The listing builds one solid part. Answer for the finished solid, in the listing's coordinates (mm). A direction names the side the tool comes from. Give positions to 0.01 mm unless a question says otherwise; leave off trailing zeros. Loops run counter-clockwise (first coordinate to the right, second up) from the corner with the lowest first, then second, coordinate; pieces in that order, holes last. Notation, with made-up numbers: M 63.5,-14.5 L 76.5,-14.5 A7 cw 76.5,-10.5 Z; hole C 14.5,61 d3. An arc over 180 degrees is marked long. Use one line per item in the form item = value. Start each with the question number.
1. The part is cut by section A-A (x = 0). Write down the section's boundary in (y, z), and give its area (3 significant figures).
2. This flat-tipped pin is pushed along its axis until it touches: pin 1 Ø2 at (x, z) = (0, 0) entering from +Y. Where does it stop, or does it pass through?
3. The part is cut by section D-D (x = -1.5). Write down the section's boundary in (y, z), and give its area (3 significant figures).
4. Straight lines are drawn through the part: line 1 (Z direction, x = 0, y = 0.7); line 2 (Y direction, x = 0.5, z = 3); line 3 (Z direction, x = -1, y = 1.45). For each, find the intervals that lie inside material, in ascending order. Write a range as from..to.
5. The mould has two halves that part along X. Classify faces 3 (the face through (-1, 1, 0)), 4 (the face through (-5.5, 1.5, -0.1)), 5 (the face through (0, 0, -1)): released by +X, released by -X, zero draft, split by the parting line, or undercut.
6. The part is cut by section C-C (y = 0.65). Write down the section's boundary in (x, z), and give its area (3 significant figures).
7. For faces 1 (the face through (0, 1, -5)), 2 (the face through (-2.373, 2.014, -3.095)), determine the directions among +Z, -Z, +X, -X, +Y, -Y from which every point of the face is accessible in a straight line to the end or side of a thin tool.
8. The part is cut by section B-B (z = 0.5). Write down the section's boundary in (x, y), and give its area (3 significant figures).
from build123d import *

# Parameters (mm, degrees)
SKETCH_1_R          = 5
EXTRUDE_1_DEPTH     = 3
SKETCH_2_R          = 3.9
CUT_EXTRUDE_1_DEPTH = 2
SKETCH_3_R          = 0.75
CUT_EXTRUDE_2_DEPTH = 8.697402159


with BuildPart() as part:
    # 草图1 → 凸台-拉伸1 (new body)
    with BuildSketch(Plane(origin=(0, 0, 0), x_dir=(1, 0, 0), z_dir=(0, 1, 0))):
        with BuildLine():
            ThreePointArc((-2.291287847, 5), (-5.5, 0), (-2.291287847, -5))
            Line((-2.291287847, -5), (0, -5))
            ThreePointArc((0, -5), (-5, 0), (0, 5))
            Line((0, 5), (-2.291287847, 5))
        make_face()
        with BuildLine():
            ThreePointArc((5, 0), (3.535533906, -3.535533906), (0, -5))
            Line((0, -5), (2.291287847, -5))
            ThreePointArc((2.291287847, -5), (4.628827236, -2.970514841), (5.5, 0))
            ThreePointArc((5.5, 0), (4.628827236, 2.970514841), (2.291287847, 5))
            Line((2.291287847, 5), (0, 5))
            ThreePointArc((0, 5), (3.535533906, 3.535533906), (5, 0))
        make_face()
        Circle(SKETCH_1_R)
    extrude(amount=EXTRUDE_1_DEPTH)

    # 草图2 → 切除-拉伸1 (cut)
    with BuildSketch(Plane(origin=(0, 3, 0), x_dir=(1, 0, 0), z_dir=(0, 1, 0))):
        with Locations(Location((0, 0, 0), (0, 0, 270))):
            Circle(SKETCH_2_R)
    extrude(amount=-CUT_EXTRUDE_1_DEPTH, mode=Mode.SUBTRACT)

    # 草图3 → 切除-拉伸2 (cut, through all)
    with BuildSketch(Plane(origin=(0, 1, 0), x_dir=(-1, 0, 0), z_dir=(0, -1, 0))):
        with Locations(Location((0, 0, 0), (0, 0, 90))):
            Circle(SKETCH_3_R)
    extrude(amount=CUT_EXTRUDE_2_DEPTH, mode=Mode.SUBTRACT)


solid = part.part
Derived:
q1.outline = M 0,-5 L 3,-5 L 3,-3.9 L 1,-3.9 L 1,-0.75 L 0,-0.75 Z; M 0,0.75 L 1,0.75 L 1,3.9 L 3,3.9 L 3,5 L 0,5 Z
q1.area = 12.9 mm2
q2.pin_1 = 1
q3.outline = M 0,-5 L 3,-5 L 3,-3.6 L 1,-3.6 L 1,3.6 L 3,3.6 L 3,5 L 0,5 Z
q3.area = 15.6 mm2
q4.line_1 = -5..-0.75, 0.75..5
q4.line_2 = 0..1
q4.line_3 = -5..-3.77, 3.77..5
q5.face_3 = undercut
q5.face_4 = released by -X
q5.face_5 = zero draft
q6.outline = M -2.29,-5 L 2.29,-5 A5.5 ccw 2.29,5 L -2.29,5 A5.5 ccw Z; hole C 0,0 d1.5
q6.area = 90.2 mm2
q7.face_1 = -Z, +X, -X, +Y, -Y
q7.face_2 = +Y
q8.outline = M -5.48,0 L -0.56,0 L -0.56,1 L -3.87,1 L -3.87,3 L -5.48,3 Z; M 0.56,0 L 5.48,0 L 5.48,3 L 3.87,3 L 3.87,1 L 0.56,1 Z
q8.area = 16.3 mm2
